The listing builds one solid part. Answer for the finished solid, in the listing's coordinates (mm). Face numbers are marked on the shaded views. A direction names the side the tool comes from. Round coordinates to 2 decimals unless told otherwise and drop trailing zeros. Order: outer loops, then holes, each group sorted by start corner. A loop starts at its lowest first (then second) coordinate and runs counter-clockwise, first axis right, second up. Notation, with made-up numbers: M 18.25,13.25 L 56.25,13.25 A13 cw 56.25,31.25 Z; hole C -10,39.25 d9. An arc over 180 degrees is marked long. Write item = value, one per line. Start each with the question number.
(1) A cutting plane is placed at D-D, the plane z = 20.5. Determine the outline of the cut face in (x, y), and give its area (3 significant figures).
(2) A cutting plane is placed at C-C, the plane y = -1. Determine the outline of the cut face in (x, z), and give its area (3 significant figures).
(3) Straight lines are drawn through the part: probe 1 along X at (y, z) = (1.75, 36.5); probe 2 along X at (y, z) = (-25.5, 19.5); probe 3 along X at (y, z) = (3, 29.5). For each, find the intervals that lie inside material, in ascending order. Write a range as from..to.
(4) A cutting plane is placed at B-B, the plane z = 36.5. Determine the outline of the cut face in (x, y).
(5) A cutting plane is placed at A-A, the plane x = 8. Determine the outline of the cut face in (y, z).
(6) Each of these flat-tipped pins is pushed along its axis until it touches: pin 1 (10.5 mm diameter, centred on x = 8, z = 36.5, fed in from -Y); pin 2 (10.5 mm diameter, centred on y = -13.5, z = 31.5, fed in from -X); pin 3 (10 mm diameter, centred on x = 54.5, z = 26, fed in from +Y). Where does it stop, or does it pass through?
(7) Which of the six approach directions +Z, -Z, +X, -X, +Y, -Y give full straight-line access (tool end or side, diameter ignored) to the marked faces 1, 2 and 3?
(8) For a pull along X with two mould halves and no side action, classify the marked faces 4, 5 and 6 as released by +X, released by -X, zero draft, split by the parting line, or undercut.
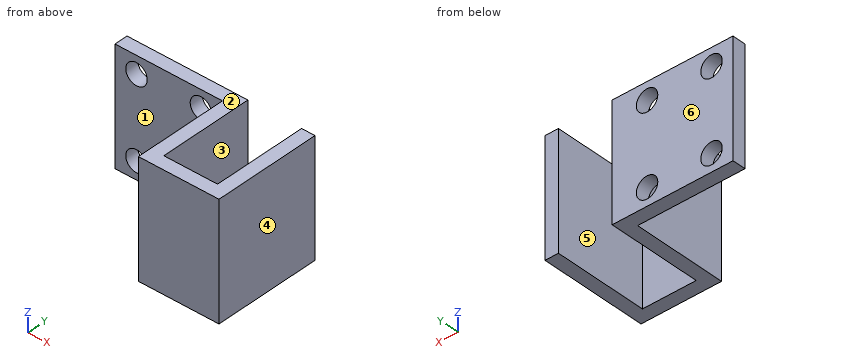
from build123d import *

# Parameters (mm, degrees)
BOSS_EXTRUDE1_DEPTH = 43
SKETCH2_R           = 4
CUT_EXTRUDE2_DEPTH  = 10


with BuildPart() as part:
    # Sketch1 → Boss-Extrude1 (new body)
    with BuildSketch(Plane.XY):
        Polygon((0, 0), (40, 0), (40, -35), (70, -35), (70, 5), (65, 5), (65, -30), (45, -30), (45, 5), (0, 5), align=None)
    extrude(amount=BOSS_EXTRUDE1_DEPTH)

    # Sketch2 → Cut-Extrude2 (cut)
    with BuildSketch(Plane.XZ):
        with Locations(Location((8, 36.5, 0), (0, 0, 270))):
            Circle(SKETCH2_R)
        with Locations(Location((32, 36.5, 0), (0, 0, 270))):
            Circle(SKETCH2_R)
        with Locations(Location((32, 6.5, 0), (0, 0, 270))):
            Circle(SKETCH2_R)
        with Locations(Location((8, 6.5, 0), (0, 0, 270))):
            Circle(SKETCH2_R)
    extrude(amount=-CUT_EXTRUDE2_DEPTH, mode=Mode.SUBTRACT)


solid = part.part
Reported:
q1.outline = M 0,0 L 40,0 L 40,-35 L 70,-35 L 70,5 L 65,5 L 65,-30 L 45,-30 L 45,5 L 0,5 Z
q1.area = 700 mm²
q2.outline = M 40,0 L 45,0 L 45,43 L 40,43 Z; M 65,0 L 70,0 L 70,43 L 65,43 Z
q2.area = 430 mm²
q3.probe_1 = 0..4, 12..28, 36..45, 65..70
q3.probe_2 = 40..45, 65..70
q3.probe_3 = 0..45, 65..70
q4.outline = M 0,0 L 4,0 L 4,5 L 0,5 Z; M 12,0 L 28,0 L 28,5 L 12,5 Z; M 36,0 L 40,0 L 40,-35 L 70,-35 L 70,5 L 65,5 L 65,-30 L 45,-30 L 45,5 L 36,5 Z
q5.outline = M 0,0 L 5,0 L 5,2.5 L 0,2.5 Z; M 0,10.5 L 5,10.5 L 5,32.5 L 0,32.5 Z; M 0,40.5 L 5,40.5 L 5,43 L 0,43 Z
q6.pin_1 = 0
q6.pin_2 = 40
q6.pin_3 = -30
q7.face_1 = +Z, -Z, -X, -Y
q7.face_2 = +Z, +X, -X, +Y, -Y
q7.face_3 = +Z, -Z, +Y
q8.face_4 = released by +X
q8.face_5 = undercut
q8.face_6 = zero draft
